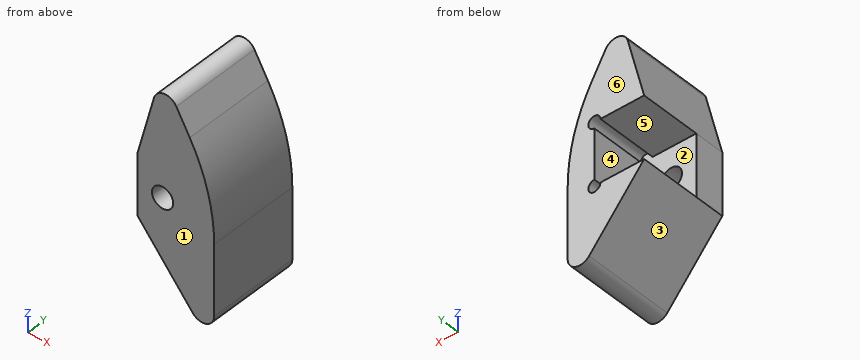
```python
from build123d import *

# Parameters (mm, degrees)
SKETCH_1_W          = 8.2
SKETCH_1_H          = 10.2
SKETCH_1_R          = 1.75
EXTRUDE_1_DEPTH     = 15
SKETCH_2_W          = 8.2
SKETCH_2_H          = 10.2
CUT_EXTRUDE_1_DEPTH = 10
SKETCH_4_R          = 1
CUT_EXTRUDE_2_DEPTH = 10
FILLET_1_R          = 30
FILLET_2_R          = 2


with BuildPart() as part:
    # ｽｹｯﾁ1 → ﾎﾞｽ - 押し出し1 (new body)
    # profile 1 of 2: a face of its own
    with BuildSketch(Plane(origin=(0, 0, 0), x_dir=(1, 0, 0), z_dir=(0, 1, 0))):
        Polygon((-0.160254038, -20), (-4.1, -5.1), (4.1, -5.1), (4.1, 5.1), (-4.1, 5.1), (8.5, 20.1), (8.5, -5), align=None)
    # profile 2 of 2: a face of its own
    with BuildSketch(Plane(origin=(0, 0, 0), x_dir=(1, 0, 0), z_dir=(0, 1, 0))):
        Rectangle(SKETCH_1_W, SKETCH_1_H)
        with Locations(Location((0, 0, 0), (0, 0, 270))):
            Circle(SKETCH_1_R, mode=Mode.SUBTRACT)
    extrude(amount=EXTRUDE_1_DEPTH)

    # ｽｹｯﾁ2 → ｶｯﾄ - 押し出し1 (cut)
    with BuildSketch(Plane(origin=(0, 15, 0), x_dir=(1, 0, 0), z_dir=(0, 1, 0))):
        Rectangle(SKETCH_2_W, SKETCH_2_H)
    extrude(amount=-CUT_EXTRUDE_1_DEPTH, mode=Mode.SUBTRACT)

    # ｽｹｯﾁ4 → ｶｯﾄ - 押し出し2 (cut)
    with BuildSketch(Plane(origin=(0, 15, 0), x_dir=(1, 0, 0), z_dir=(0, 1, 0))):
        with Locations((4.1, 5.1)):
            Circle(SKETCH_4_R)
        with Locations((4.1, -5.1)):
            Circle(SKETCH_4_R)
    extrude(amount=-CUT_EXTRUDE_2_DEPTH, mode=Mode.SUBTRACT)

    # ﾌｨﾚｯﾄ1
    fillet_1_edges = [part.edges().sort_by_distance(p)[0] for p in [
        (8.5, 7.5, 5),
    ]]
    fillet(fillet_1_edges, radius=FILLET_1_R)

    # ﾌｨﾚｯﾄ2
    fillet_2_edges = [part.edges().sort_by_distance(p)[0] for p in [
        (8.5, 7.5, -20.1),
        (-0.160254038, 7.5, 20),
    ]]
    fillet(fillet_2_edges, radius=FILLET_2_R)


solid = part.part
```
Build history of the part. All positions in model axes, mm. Face numbers are marked on the shaded views. A direction names the side the tool comes from. Give positions to 0.01 mm unless a question says otherwise; leave off trailing zeros. Loops run counter-clockwise (first coordinate to the right, second up) from the corner with the lowest first, then second, coordinate; pieces in that order, holes last. Notation, with made-up numbers: (49, 82) -> (105, 82) arc R31 ccw to (105, 111) -> close; hole circle Ø8 at (-0.5, 17). An arc over 180 degrees is marked (long way). One line per question, with ' | ' between items.
Q1. Cut at A-A, the plane y = 1.25. Write the cut outline in (x, z).
Filled sheet:
outline: (-4.1, -5.1) -> (4.97, -15.9) arc R2 ccw to (8.5, -14.61) -> (8.5, -3.04) arc R30 ccw to (4.48, 11.96) -> (2.27, 15.8) arc R2 ccw to (-1.4, 15.31) -> (-4.1, 5.1) -> close; hole circle Ø3.5 at (0, 0)
Q2. Cut at B-B, the plane y = 12. Write the cut outline in (x, z), plus the area to 3 significant figures.
Filled sheet:
outline: (-4.1, -5.1) -> (4.97, -15.9) arc R2 ccw to (8.5, -14.61) -> (8.5, -3.04) arc R30 ccw to (4.48, 11.96) -> (2.27, 15.8) arc R2 ccw to (-1.4, 15.31) -> (-4.1, 5.1) -> (3.1, 5.1) arc R1 cw (long way) to (4.1, 4.1) -> (4.1, -4.1) arc R1 cw (long way) to (3.1, -5.1) -> close | area: 211 mm²
Q3. Tool access for the marked faces 5 and 6: list every direction of +Z, -Z, +X, -X, +Y, -Y with a clear straight run to the whole face (end or side of a thin tool).
Filled sheet:
face 5: -X, +Y | face 6: +Z, -Z, +X, -X, +Y
Q4. Pull direction Z, two halves, no side cores. Call the marked faces 1, 2, 3 and 4: pulls with the +Z half, pulls with the -Z half, needs draft (parallel to the pull), parting line crosses it, or undercut.
Filled sheet:
face 1: needs draft | face 2: undercut | face 3: pulls with the -Z half | face 4: undercut
Q5. Cut at C-C, the plane z = 0. Write the cut outline in (x, y).
Filled sheet:
outline: (-4.1, 0) -> (-1.75, 0) -> (-1.75, 5) -> (-4.1, 5) -> close; (1.75, 0) -> (8.35, 0) -> (8.35, 15) -> (4.1, 15) -> (4.1, 5) -> (1.75, 5) -> close
Q6. Cut at D-D, the plane x = 0. Write the cut outline in (y, z).
Filled sheet:
outline: (0, -9.98) -> (15, -9.98) -> (15, -5.1) -> (5, -5.1) -> (5, -1.75) -> (0, -1.75) -> close; (0, 1.75) -> (5, 1.75) -> (5, 5.1) -> (15, 5.1) -> (15, 16.73) -> (0, 16.73) -> close
Q7. Drop flat-ended pins along their axis: pin 1 (2 mm diameter, centred on x = -0.5, y = 12, fed in from -Z); pin 2 (2 mm diameter, centred on x = 4, y = 11.5, fed in from +Z); pin 3 (3 mm diameter, centred on x = -2.5, y = 8, fed in from +Z). Give the stop position or say it passes through.
Filled sheet:
pin 1: stops at z = -10.58 | pin 2: stops at z = 14.53 | pin 3: stops at z = 16.08
Q8. Drill centre lines: line 1 along Z through (x, y) = (0, 3.35); line 2 along X through (y, z) = (1.7, 0); line 3 along Y through (x, z) = (3.25, 5). Where is each one in solid material? Low to high. Write a range as [from, to].
Filled sheet:
line 1: z = [-9.98, -1.75], [1.75, 16.73] | line 2: x = [-4.1, -1.75], [1.75, 8.35] | line 3: y = [0, 5]
